Work out the finished part from the listing and answer in its coordinate system (mm). Face numbers are marked on the shaded views. A direction names the side the tool comes from. Coordinates: 2 decimals unless noted, no trailing zeros. Loops run counter-clockwise (first coordinate to the right, second up) from the corner with the lowest first, then second, coordinate; pieces in that order, holes last. Notation, with made-up numbers: (-23.75, 39) -> (29.25, 39) arc R22 cw to (29.25, 56) -> close; hole circle Ø9 at (-19, -38). An arc over 180 degrees is marked (long way). Use a Markdown table: item, result.
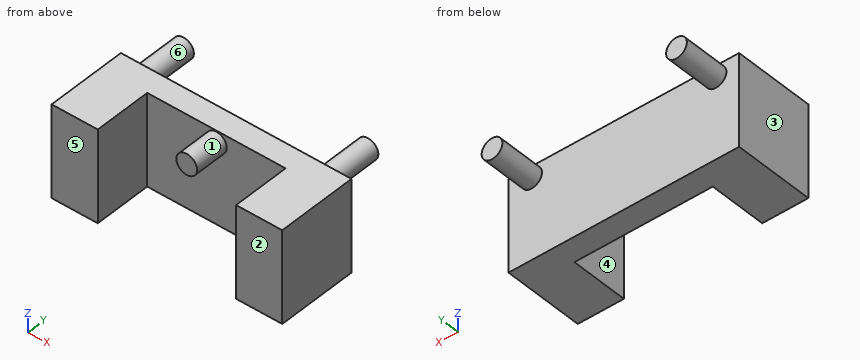
from build123d import *

# Parameters (mm, degrees)
SKETCH1_W                = 25.4
SKETCH1_H                = 10.16
BOSS_EXTRUDE1_DEPTH      = 8.89
SKETCH2_W                = 15.24
SKETCH2_H                = 10.16
CUT_EXTRUDE1_DEPTH       = 7.62
BOSS_EXTRUDE2_DEPTH      = 5.08
BOSS_EXTRUDE2_DEPTH_BACK = 5.08
SKETCH3_R                = 1.143
SKETCH3_5_R              = 1.143
BOSS_EXTRUDE3_DEPTH      = 6.35


with BuildPart() as part:
    # Sketch1 → Boss-Extrude1 (new body)
    with BuildSketch(Plane(origin=(0, 0, 0), x_dir=(1, 0, 0), z_dir=(0, 1, 0))):
        with Locations((12.7, -5.08)):
            Rectangle(SKETCH1_W, SKETCH1_H)
    extrude(amount=BOSS_EXTRUDE1_DEPTH)

    # Sketch2 → Cut-Extrude1 (cut)
    with BuildSketch(Plane(origin=(0, 6.35, 0), x_dir=(1, 0, 0), z_dir=(0, 1, 0))):
        with Locations((12.7, -5.08)):
            Rectangle(SKETCH2_W, SKETCH2_H)
    extrude(amount=-CUT_EXTRUDE1_DEPTH, mode=Mode.SUBTRACT)

    # Sketch3 → Boss-Extrude2 (add, two sides: drawn at the far end of the back side and taken through both)
    with BuildSketch(Plane(origin=(0, 8.89, 0), x_dir=(1, 0, 0), z_dir=(0, 1, 0)).offset(-BOSS_EXTRUDE2_DEPTH_BACK)):
        with Locations(Location((2.54, -8.89, 0), (0, 0, 270))):
            Circle(SKETCH3_R)
        with Locations(Location((22.86, -8.89, 0), (0, 0, 270))):
            Circle(SKETCH3_R)
    extrude(amount=BOSS_EXTRUDE2_DEPTH + BOSS_EXTRUDE2_DEPTH_BACK)

    # Sketch3_5 → Boss-Extrude3 (add)
    with BuildSketch(Plane(origin=(0, 8.89, 0), x_dir=(1, 0, 0), z_dir=(0, 1, 0))):
        with Locations(Location((12.7, -8.89, 0), (0, 0, 270))):
            Circle(SKETCH3_5_R)
    extrude(amount=-BOSS_EXTRUDE3_DEPTH)


solid = part.part
Q1. For the marked faces 4, 5 and 6, determine the directions among +Z, -Z, +X, -X, +Y, -Y from which every point of the face is accessible in a straight line to the end or side of a thin tool.
Solved:
| item | result |
|---|---|
| face 4 | +Z, -Z, -Y |
| face 5 | +Z, -Z, +X, -X, -Y |
| face 6 | +Y |
Q2. Consider line 1 (X direction, y = 6, z = 3.75); line 2 (Y direction, x = 4.25, z = 8.75); line 3 (Y direction, x = 17.5, z = 9.75). Determine where each line is inside the solid, lowest interval first. Write a range as [from, to].
Solved:
| item | result |
|---|---|
| line 1 | [0, 5.08], [20.32, 25.4] |
| line 2 | [0, 8.89] |
| line 3 | [6.35, 8.89] |
Q3. Section C-C on z = 8.89 is taken. Determine the outline of the cut face in (x, y), and give its area (3 significant figures).
Solved:
| item | result |
|---|---|
| outline | (0, 0) -> (5.08, 0) -> (5.08, 6.35) -> (11.56, 6.35) -> (11.56, 2.54) -> (13.84, 2.54) -> (13.84, 6.35) -> (20.32, 6.35) -> (20.32, 0) -> (25.4, 0) -> (25.4, 8.89) -> (24, 8.89) -> (24, 13.97) -> (21.72, 13.97) -> (21.72, 8.89) -> (3.68, 8.89) -> (3.68, 13.97) -> (1.4, 13.97) -> (1.4, 8.89) -> (0, 8.89) -> close |
| area | 161 mm² |
Q4. Determine the mould class of the marked faces 1, 2 and 3 for opening direction X: pulls with the +X half, pulls with the -X half, needs draft (parallel to the pull), parting line crosses it, or undercut.
Solved:
| item | result |
|---|---|
| face 1 | undercut |
| face 2 | needs draft |
| face 3 | pulls with the -X half |
Q5. Section B-B on x = 12.7 is taken. Determine the outline of the cut face in (y, z), and give its area (3 significant figures).
Solved:
| item | result |
|---|---|
| outline | (2.54, 7.75) -> (6.35, 7.75) -> (6.35, 0) -> (8.89, 0) -> (8.89, 10.16) -> (6.35, 10.16) -> (6.35, 10.03) -> (2.54, 10.03) -> close |
| area | 34.5 mm² |
Q6. Section D-D on y = 11.25 is taken. Determine the outline of the cut face in (x, z), and give its area (3 significant figures).
Solved:
| item | result |
|---|---|
| outline | circle Ø2.29 at (2.54, 8.89); circle Ø2.29 at (22.86, 8.89) |
| area | 8.21 mm² |
Q7. Section A-A on y = 1.25 is taken. Determine the outline of the cut face in (x, z).
Solved:
| item | result |
|---|---|
| outline | (0, 0) -> (5.08, 0) -> (5.08, 10.16) -> (0, 10.16) -> close; (20.32, 0) -> (25.4, 0) -> (25.4, 10.16) -> (20.32, 10.16) -> close |
Q8. Given pin 1 Ø1.5 at (x, z) = (15, 4) entering from -Y; pin 2 Ø3 at (x, z) = (8.5, 7) entering from +Y; pin 3 Ø4 at (y, z) = (11, 2.5) entering from -X; pin 4 Ø6 at (x, z) = (10, 7.5) entering from -Y, each flat-ended and moving along its own axis, determine where each tip first touches the part or whether it passes through.
Solved:
| item | result |
|---|---|
| pin 1 | y = 6.35 |
| pin 2 | y = 8.89 |
| pin 3 | through |
| pin 4 | y = 2.54 |
